from build123d import *

# Parameters (mm, degrees)
SKETCH2_R           = 16.5
BOSS_EXTRUDE1_DEPTH = 0.75
SKETCH3_R           = 15.5
SKETCH3_R_2         = 15
BOSS_EXTRUDE2_DEPTH = 1.5
CHAMFER1_SIZE       = 0.75


with BuildPart() as part:
    # Sketch2 → Boss-Extrude1 (new body)
    with BuildSketch(Plane(origin=(0, 0, 0), x_dir=(1, 0, 0), z_dir=(0, 1, 0))):
        with Locations(Location((0, 0, 0), (0, 0, 270))):
            Circle(SKETCH2_R)
    extrude(amount=BOSS_EXTRUDE1_DEPTH)

    # Sketch3 → Boss-Extrude2 (add)
    with BuildSketch(Plane(origin=(0, 0.75, 0), x_dir=(1, 0, 0), z_dir=(0, 1, 0))):
        with Locations(Location((0, 0, 0), (0, 0, 270))):
            Circle(SKETCH3_R)
        with Locations(Location((0, 0, 0), (0, 0, 270))):
            Circle(SKETCH3_R_2, mode=Mode.SUBTRACT)
    extrude(amount=BOSS_EXTRUDE2_DEPTH)

    # Chamfer1
    chamfer1_edges = [part.edges().sort_by_distance(p)[0] for p in [
        (0, 0, -16.5),
    ]]
    chamfer(chamfer1_edges, length=CHAMFER1_SIZE - 0.0001)  # a hair under: the kernel refuses the full size


solid = part.part
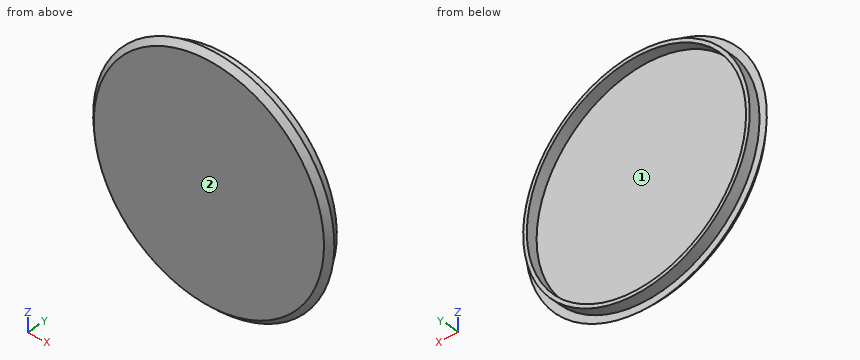
Geometry: final body of the model. Coordinates: model frame, mm. Face numbers are marked on the shaded views. Coordinates: 2 decimals unless noted, no trailing zeros. Write each loop counter-clockwise with the first axis right and the second up, starting at its lowest first coordinate (ties: lowest second). Pieces come first, ordered by that corner, then holes. Notation, with made-up numbers: (67, -32) - (82, -32) arc R28 cw to (82, -13) - close; hole circle Ø3 at (11.25, -35). An arc over 180 degrees is marked (long way). Return JSON: item names as keys, results as strings.
Item 1: Section query B-B (y = 1.85). Output: boundary loops of the cut face in (x, z), and give its area (3 significant figures).
Completed:
{"outline": "circle Ø31 at (0, 0); hole circle Ø30 at (0, 0)", "area": "47.9 mm2"}
Item 2: Pull-direction query (X, two-part tool) for the marked faces 1 and 2; classes: +X half, -X half, draft (parallel to the pull), parting line (faces both ways), or undercut.
Completed:
{"face 1": "undercut", "face 2": "draft"}
Item 3: Line query: L1, parallel to X at y = 1.25, z = 0; L2, parallel to Y at x = -12.5, z = -7; L3, parallel to X at y = 1.3, z = 4. Output: solid intervals per line, ascending.
Completed:
{"L1": "x = -15.5 to -15, 15 to 15.5", "L2": "y = 0 to 0.75", "L3": "x = -14.97 to -14.46, 14.46 to 14.97"}
Item 4: Pin query (flat end, axial travel): pin 1 Ø4 at (x, z) = (9.5, -6.5) entering from +Y. Return the tip coordinate at first contact, or that it passes through.
Completed:
{"pin 1": "stops at y = 0.75"}
